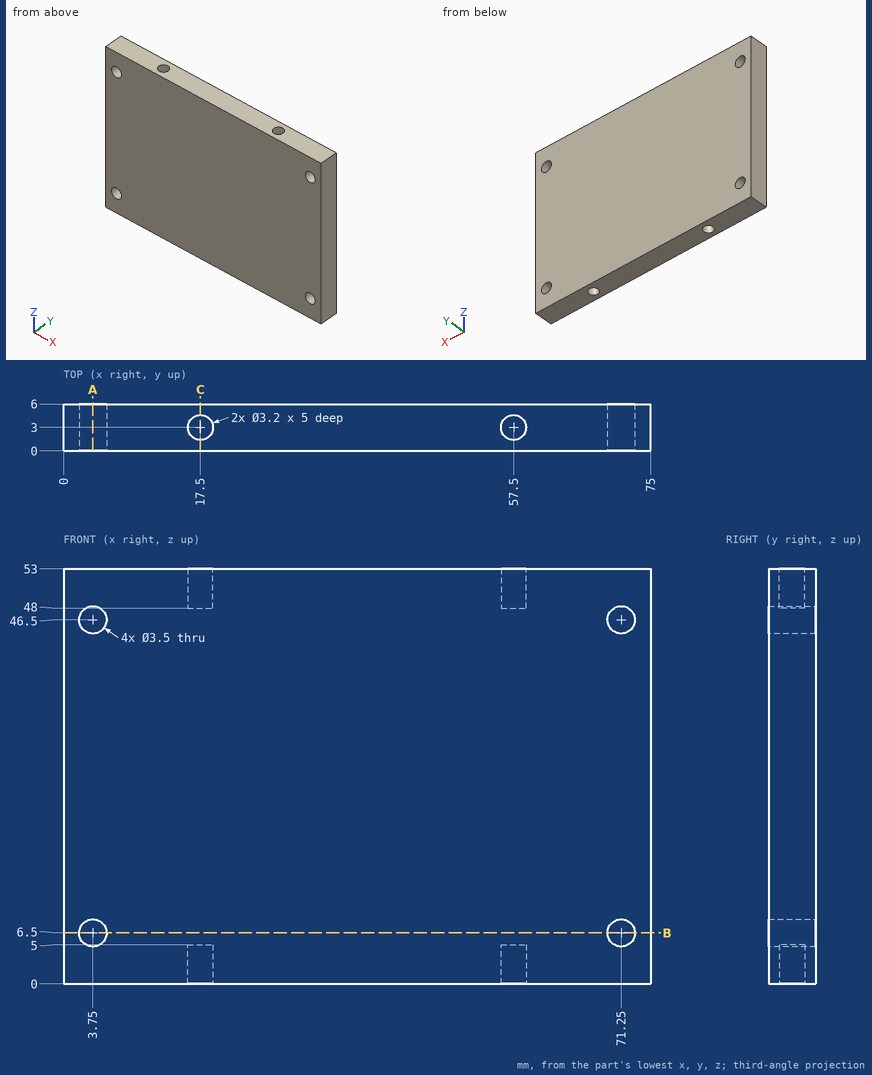
Can you work these out from the drawing? Everything is in mm from the part's minimum corner. Coordinates: 2 decimals unless noted, no trailing zeros. Order: outer loops, then holes, each group sorted by start corner. A loop starts at its lowest first (then second) coordinate and runs counter-clockwise, first axis right, second up. Notation, with made-up numbers: M 78,67.25 L 104,67.25 A20 cw 104,86.25 Z; hole C 16,-18.5 d2. An arc over 180 degrees is marked long. Answer as CSV lines item,"result". Start each with the question number.
1. For pin 1 (1.9 mm diameter, centred on x = 57.5, y = 3, fed in from +Z); pin 2 (3.5 mm diameter, centred on x = 17.5, y = 2.5, fed in from -Z), each with a flat end and sliding along its axis, tell me the tip position at first contact or that it passes through.
2. I want a section at C-C, the plane x = 17.5. Write out the boundary of the cut face in (y, z), and give its area (3 significant figures).
3. I want a section at A-A, the plane x = 3.75. Write out the boundary of the cut face in (y, z).
4. I need wall thicknesses on line 1 (X direction, y = 1.8, z = 6.5); line 2 (Z direction, x = 71, y = 1.8); line 3 (Y direction, x = 57, z = 50). Which ranges of each line are inside material? Lowest first, please. Write a range as [from, to].
5. I want a section at B-B, the plane z = 6.5. Write out the boundary of the cut face in (x, y).
Recorded:
1,pin 1,"stops at z = 48"
1,pin 2,"stops at z = 0"
2,outline,"M 0,0 L 1.4,0 L 1.4,5 L 4.6,5 L 4.6,0 L 6,0 L 6,53 L 4.6,53 L 4.6,48 L 1.4,48 L 1.4,53 L 0,53 Z"
2,area,"286 mm2"
3,outline,"M 0,0 L 6,0 L 6,4.75 L 0,4.75 Z; M 0,8.25 L 6,8.25 L 6,44.75 L 0,44.75 Z; M 0,48.25 L 6,48.25 L 6,53 L 0,53 Z"
4,line 1,"x = [0, 2], [5.5, 69.5], [73, 75]"
4,line 2,"z = [0, 4.77], [8.23, 44.77], [48.23, 53]"
4,line 3,"y = [0, 1.48], [4.52, 6]"
5,outline,"M 0,0 L 2,0 L 2,6 L 0,6 Z; M 5.5,0 L 69.5,0 L 69.5,6 L 5.5,6 Z; M 73,0 L 75,0 L 75,6 L 73,6 Z"
